from build123d import *

# Parameters (mm, degrees)
F0_W     = 100
F0_H     = 50
F0_R     = 3
F1_DEPTH = 5
F2_DEPTH = 10


with BuildPart() as f1:
    # F0 (on Front) → F1 (new body)
    with BuildSketch(Plane.XZ):
        Rectangle(F0_W, F0_H)
        Circle(F0_R, mode=Mode.SUBTRACT)
        Circle(F0_R)
    extrude(amount=F1_DEPTH)

    # F0 (on Front) → F2 (join)
    with BuildSketch(Plane.XZ):
        Circle(F0_R)
    extrude(amount=F2_DEPTH)


solid = f1.part
Check sheet for the modelled part. Datum: model origin and axes. Units: mm. A direction names the side the tool comes from. Give positions to 0.01 mm unless a question says otherwise; leave off trailing zeros. Write each loop counter-clockwise with the first axis right and the second up, starting at its lowest first coordinate (ties: lowest second). Pieces come first, ordered by that corner, then holes. Notation, with made-up numbers: (-21, -25.5) -> (-9, -25.5) arc R30 ccw to (-9, 4.5) -> close; hole circle Ø8 at (28, 8.5). An arc over 180 degrees is marked (long way). One line per item, written item: value. Start each with the question number.
Item 1: Tool access check on faces 1 (the cylindrical face through (-3, -7, 0)), 2 (the flat face through (50, -2, 0)). Record the directions out of +Z, -Z, +X, -X, +Y, -Y that give a thin tool (end or side, any length) a straight path to the whole face; none if there is none.
Item 2: Material ranges on probe 1 along Y at (x, z) = (-21.5, -9); probe 2 along X at (y, z) = (-8.5, -0.5), recorded low to high. Write a range as from..to.
Item 3: Section check B-B on x = 0. Record the cut outline in (y, z).
Item 4: Section check A-A on z = 0. Record the cut outline in (x, y).
Item 5: Gauge pin test, flat ends, axial feed: pin 1 (15 mm diameter, centred on x = -8.5, z = -7, fed in from -Y); pin 2 (3 mm diameter, centred on y = -7, z = 5, fed in from +X). Record the tip position at first contact, or that the pin passes through.
Item 6: Section check D-D on z = 16. Record the cut outline in (x, y).
Item 7: Section check C-C on y = -8. Record the cut outline in (x, z).
Results list:
1. face 1: -Y
1. face 2: +Z, -Z, +X, +Y, -Y
2. probe 1: -5..0
2. probe 2: -2.96..2.96
3. outline: (-10, -3) -> (-5, -3) -> (-5, -25) -> (0, -25) -> (0, 25) -> (-5, 25) -> (-5, 3) -> (-10, 3) -> close
4. outline: (-50, -5) -> (-3, -5) -> (-3, -10) -> (3, -10) -> (3, -5) -> (50, -5) -> (50, 0) -> (-50, 0) -> close
5. pin 1: y = -5
5. pin 2: through
6. outline: (-50, -5) -> (50, -5) -> (50, 0) -> (-50, 0) -> close
7. outline: circle Ø6 at (0, 0)
